```python
from build123d import *

# Parameters (mm, degrees)
SKETCH004_W      = 30
SKETCH004_H      = 50
EXTRUDE003_DEPTH = 20
SKETCH002_R      = 6.95
EXTRUDE001_DEPTH = 12.5
SKETCH001_R      = 7
EXTRUDE_DEPTH    = 15
SKETCH003_W      = 7
SKETCH003_H      = 7
EXTRUDE002_DEPTH = 2.5
FILLET_R         = 1


with BuildPart() as extrude003:
    # Sketch004 → Extrude003 (new body)
    with BuildSketch(Plane.XZ):
        Rectangle(SKETCH004_W, SKETCH004_H)
    extrude(amount=EXTRUDE003_DEPTH)


with BuildPart() as extrude001:
    # Sketch002 → Extrude001 (new body)
    with BuildSketch(Plane.XY.offset(8)):
        Circle(SKETCH002_R)
    extrude(amount=EXTRUDE001_DEPTH)


with BuildPart() as extrude_body:
    # Sketch001 → Extrude (new body, symmetric)
    with BuildSketch(Plane.XZ):
        Circle(SKETCH001_R)
    extrude(amount=EXTRUDE_DEPTH, both=True)


with BuildPart() as cut:
    # Sketch → Revolve (revolve)
    with BuildSketch(Plane.XZ):
        with BuildLine():
            ThreePointArc((0, -12.95), (12.95, 0), (0, 12.95))
            Line((0, 12.95), (0, -12.95))
        make_face()
    revolve(axis=Axis((0, 0, 0), (0, 0, 1)))

    # Cut: cut Extrude body
    add(extrude_body.part, mode=Mode.SUBTRACT)


with BuildPart() as cut001:
    # Sketch003 (on Face3 of Extrude001) → Extrude002 (new body)
    with BuildSketch(Plane.XY.offset(20.5)):
        Rectangle(SKETCH003_W, SKETCH003_H)
    extrude(amount=EXTRUDE002_DEPTH)

    # Fillet
    fillet_edges = [cut001.edges().sort_by_distance(p)[0] for p in [
        (-3.5, -3.5, 21.75),
        (3.5, -3.5, 21.75),
        (3.5, 3.5, 21.75),
        (-3.5, 3.5, 21.75),
    ]]
    fillet(fillet_edges, radius=FILLET_R)

    # Fusion: union Extrude001, Cut
    add(extrude001.part)
    add(cut.part)

    # Cut001: cut Extrude003
    add(extrude003.part, mode=Mode.SUBTRACT)


solid = cut001.part
```
Could you check a few things on this model? Use its own coordinates, in mm. A direction names the side the tool comes from. Coordinates: 2 decimals unless noted, no trailing zeros. Loops run counter-clockwise (first coordinate to the right, second up) from the corner with the lowest first, then second, coordinate; pieces in that order, holes last. Notation, with made-up numbers: M 4.5,53 L 29.5,53 A15 cw 29.5,77 Z; hole C 46.5,-24.5 d11. An arc over 180 degrees is marked long. Put each result on its own line as item: value. Start each with the question number.
(1) Suppose I cut it at D-D on y = 7.5. Please give me the cut outline in (x, z), then the cut area to 3 significant figures.
(2) For faces 4 (the face through (-3.215, 3.199, 21.768)), 5 (the face through (0, 4, 20.5)), 6 (the face through (3.215, 3.199, 21.768)), which set-ups out of +Z, -Z, +X, -X, +Y, -Y let a thin tool reach every point of the face, with its end or its side?
(3) Suppose I cut it at C-C on x = 6. Please give me the cut outline in (y, z), then the cut area to 3 significant figures.
(4) Thinking about a two-plate mould opening in X: for faces 1 (the face through (6.466, 5.371, -2.681)), 2 (the face through (0.15, 6.95, 15.65)), 3 (the face through (-3.5, 1, 22)), which applies, pulls with the +X half, pulls with the -X half, needs draft (parallel to the pull), parting line crosses it, or undercut?
(5) I need wall thicknesses on line 1 (Z direction, x = -5.5, y = 3); line 2 (X direction, y = 2, z = 5); line 3 (X direction, y = 7, z = 0). Which ranges of each line are inside material? Lowest first, please. Write a range as from..to.
(6) Will these pins go through, and if not, where does the flat tip stop? P1, Ø1.2, axis at y = 1, z = 22, coming from the -X side; P2, Ø0.8, axis at y = 2, z = 21.5, coming from the +X side; P3, Ø5, axis at x = 4, y = 9.5, coming from the -Z side.
(7) Suppose I cut it at B-B on z = 0. Please give me the cut outline in (x, y).
(8) Suppose I cut it at A-A on x = 0. Please give me the cut outline in (y, z), then the cut area to 3 significant figures.
Solutions:
1. outline: C 0,0 d21.11; hole C 0,0 d14
1. area: 196 mm2
2. face 4: +Z, -X, +Y
2. face 5: +Z, +Y
2. face 6: +Z, +X, +Y
3. outline: M 0,-11.48 A11.48 ccw 10.9,-3.61 L 0,-3.61 Z; M 0,3.61 L 10.9,3.61 A11.48 ccw 3.51,10.93 L 3.51,20.5 L 0,20.5 Z
3. area: 158 mm2
4. face 1: undercut
4. face 2: parting line crosses it
4. face 3: pulls with the -X half
5. line 1: z = -11.33..-4.33, 4.33..20.5
5. line 2: x = -11.78..-4.9, 4.9..11.78
5. line 3: x = -10.9..-7, 7..10.9
6. P1: stops at x = -3.5
6. P2: stops at x = 3.5
6. P3: stops at z = -10.33
7. outline: M -12.95,0 L -7,0 L -7,10.9 A12.95 ccw Z; M 7,0 L 12.95,0 A12.95 ccw 7,10.9 Z
8. outline: M 0,-12.95 A12.95 ccw 10.9,-7 L 0,-7 Z; M 0,7 L 10.9,7 A12.95 ccw 6.95,10.93 L 6.95,20.5 L 3.5,20.5 L 3.5,23 L 0,23 Z
8. area: 157 mm2
